Here's the drawing with two shaded views (mm, measured from the low corner). I have some questions. A direction names the side the tool comes from. Give positions to 0.01 mm unless a question says otherwise; leave off trailing zeros. Loops run counter-clockwise (first coordinate to the right, second up) from the corner with the lowest first, then second, coordinate; pieces in that order, holes last. Notation, with made-up numbers: (8, 20) -> (44, 20) arc R32 cw to (44, 57) -> close; hole circle Ø1 at (33.5, -38.5). An arc over 180 degrees is marked (long way). Put each result on its own line as item: value.
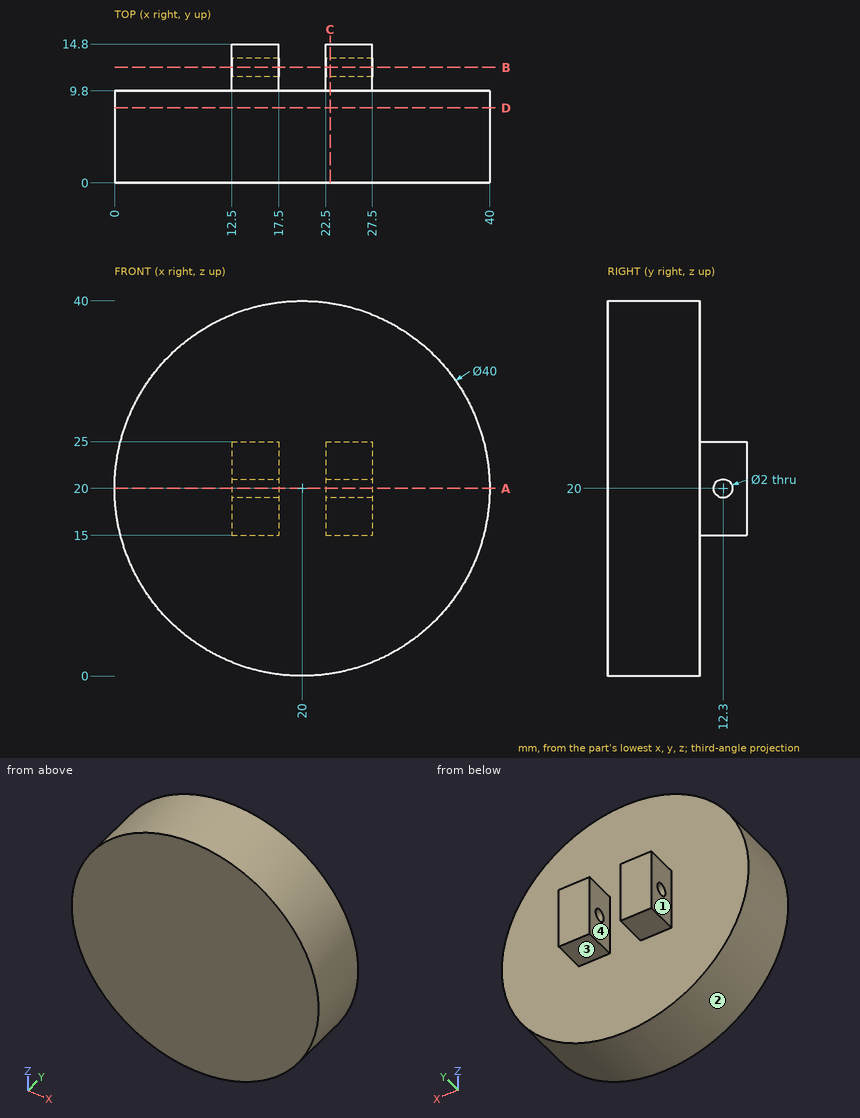
1. I'm going to push flat-ended pins straight in: pin 1 (2.5 mm diameter, centred on y = 12.5, z = 20.5, fed in from +X); pin 2 (4 mm diameter, centred on x = 14.5, y = 12.5, fed in from -Z); pin 3 (1.5 mm diameter, centred on y = 11.5, z = 21.5, fed in from -X); pin 4 (1.6 mm diameter, centred on y = 12.3, z = 20, fed in from -X). Where does each tip first touch, or does it pass through?
Recorded:
pin 1: stops at x = 27.5
pin 2: stops at z = 15
pin 3: stops at x = 12.5
pin 4: passes through
2. I need wall thicknesses on line 1 (Y direction, x = 25, z = 20); line 2 (Y direction, x = 18, z = 30); line 3 (Z direction, x = 24.5, y = 10). Which ranges of each line are inside material? Lowest first, please.
Recorded:
line 1: y = 0 to 11.3, 13.3 to 14.8
line 2: y = 0 to 9.8
line 3: z = 15 to 25
3. If we section it at C-C (x = 23): List the corners of the cut face in (y, z) for me.
Recorded:
outline: (0, 0.23) -> (9.8, 0.23) -> (9.8, 15) -> (14.8, 15) -> (14.8, 25) -> (9.8, 25) -> (9.8, 39.77) -> (0, 39.77) -> close; hole circle Ø2 at (12.3, 20)
4. For the marked faces 1, 2, 3 and 4, which set-ups out of +Z, -Z, +X, -X, +Y, -Y let a thin tool reach every point of the face, with its end or its side?
Recorded:
face 1: +Z, -Z, -X, +Y
face 2: +Y, -Y
face 3: -Z, +X, -X, +Y
face 4: +Z, -Z, +Y
5. If we section it at D-D (y = 8): List the corners of the cut face in (x, z) for me, then the cut area to 3 significant figures.
Recorded:
outline: circle Ø40 at (20, 20)
area: 1,260 mm^2
6. If we section it at A-A (z = 20): List the corners of the cut face in (x, y) for me.
Recorded:
outline: (0, 0) -> (40, 0) -> (40, 9.8) -> (27.5, 9.8) -> (27.5, 11.3) -> (22.5, 11.3) -> (22.5, 9.8) -> (17.5, 9.8) -> (17.5, 11.3) -> (12.5, 11.3) -> (12.5, 9.8) -> (0, 9.8) -> close; (12.5, 13.3) -> (17.5, 13.3) -> (17.5, 14.8) -> (12.5, 14.8) -> close; (22.5, 13.3) -> (27.5, 13.3) -> (27.5, 14.8) -> (22.5, 14.8) -> close
7. If we section it at B-B (y = 12.3): List the corners of the cut face in (x, z) for me, then the cut area to 3 significant figures.
Recorded:
outline: (12.5, 15) -> (17.5, 15) -> (17.5, 19) -> (12.5, 19) -> close; (12.5, 21) -> (17.5, 21) -> (17.5, 25) -> (12.5, 25) -> close; (22.5, 15) -> (27.5, 15) -> (27.5, 19) -> (22.5, 19) -> close; (22.5, 21) -> (27.5, 21) -> (27.5, 25) -> (22.5, 25) -> close
area: 80.0 mm^2
